from build123d import *

# Parameters (mm, degrees)
SKETCH_2_W                       = 1.5
SKETCH_2_H                       = 108.5
SM_BASE_FLANGE_1_DEPTH           = 385
SM_EDGE_FLANGE_2_STRIP_W         = 7.4732
SM_EDGE_FLANGE_2_STRIP_H         = 1.5
SM_EDGE_FLANGE_2_STRIP_CUT_DEPTH = 385
SM_EDGE_FLANGE_2_DEPTH           = 385
SKETCH_13_W                      = 19.831026495
SKETCH_13_H                      = 4.393295337
CUT_EXTRUDE_1_DEPTH              = 8
SM_EDGE_FLANGE_3_STRIP_W         = 7.4732
SM_EDGE_FLANGE_3_STRIP_H         = 1.5
SM_EDGE_FLANGE_3_STRIP_CUT_DEPTH = 385
SM_EDGE_FLANGE_3_DEPTH           = 385
SKETCH_18_W                      = 20.05650784
SKETCH_18_H                      = 5.183741357
CUT_EXTRUDE_2_DEPTH              = 8
SKETCH_19_W                      = 25.725423763
SKETCH_19_H                      = 11.342633063
CUT_EXTRUDE_3_DEPTH              = 140
SKETCH_20_W                      = 20.859346665
SKETCH_20_H                      = 6.188811882
CUT_EXTRUDE_4_DEPTH              = 15
SKETCH_21_W                      = 1.5
SKETCH_21_H                      = 153.4
EXTRUDE_1_DEPTH                  = 452.41
SKETCH_22_R                      = 2.75
CUT_EXTRUDE_5_DEPTH              = 20
SKETCH_23_R                      = 2.75
CUT_EXTRUDE_6_DEPTH              = 20
SKETCH_24_R                      = 2.75
CUT_EXTRUDE_7_DEPTH              = 20
SKETCH_28_W                      = 3.977690792
SKETCH_28_H                      = 20
CUT_EXTRUDE_8_DEPTH              = 10
SM_EDGE_FLANGE_5_STRIP_W         = 7.4732
SM_EDGE_FLANGE_5_STRIP_H         = 1.5
SM_EDGE_FLANGE_5_STRIP_CUT_DEPTH = 432.41
SM_EDGE_FLANGE_5_DEPTH           = 432.41
SKETCH_32_R                      = 2.75
CUT_EXTRUDE_9_DEPTH              = 10
CUT_EXTRUDE_START                = -2
CUT_EXTRUDE_10_DEPTH             = 2


# Read off the part's stored shape, not the designer's step: 切除-拉伸10
# Sheet-metal steps are written as plain solids
with BuildPart() as part:
    # Sketch 2 → 基体-法兰1 (new body)
    with BuildSketch(Plane.XY):
        with Locations((0.75, 54.25)):
            Rectangle(SKETCH_2_W, SKETCH_2_H)
    extrude(amount=SM_BASE_FLANGE_1_DEPTH)

    # 边线-法兰2 strip (across the edge) → 边线-法兰2 strip cut (cut)
    with BuildSketch(Plane(origin=(1.5, 0, 385), x_dir=(0, 1, 0), z_dir=(0, 0, -1))):
        with Locations((-1.5, -0.75)):
            Rectangle(SM_EDGE_FLANGE_2_STRIP_W, SM_EDGE_FLANGE_2_STRIP_H)
    extrude(amount=SM_EDGE_FLANGE_2_STRIP_CUT_DEPTH, mode=Mode.SUBTRACT)

    # 边线-法兰2 section (across the edge) → 边线-法兰2 (add)
    with BuildSketch(Plane(origin=(1.5, 0, 385), x_dir=(0, 1, 0), z_dir=(0, 0, -1))):
        with BuildLine():
            Line((0, 0.7366), (0, 13.5))
            Line((0, 13.5), (1.5, 13.5))
            Line((1.5, 13.5), (1.5, 0.7366))
            ThreePointArc((1.5, 0.7366), (1.715745145, 0.215745145), (2.2366, 0))
            Line((2.2366, 0), (2.2366, -1.5))
            ThreePointArc((2.2366, -1.5), (0.655084973, -0.844915027), (0, 0.7366))
        make_face()
    extrude(amount=SM_EDGE_FLANGE_2_DEPTH)

    # 草图13 → 切除-拉伸1 (cut)
    with BuildSketch(Plane(origin=(0, 0, 0), x_dir=(-1, 0, 0), z_dir=(0, 0, -1))):
        with Locations((-9.915513247, 0.039952332)):
            Rectangle(SKETCH_13_W, SKETCH_13_H)
    extrude(amount=-CUT_EXTRUDE_1_DEPTH, mode=Mode.SUBTRACT)

    # 边线-法兰3 strip (across the edge) → 边线-法兰3 strip cut (cut)
    with BuildSketch(Plane(origin=(1.5, 108.5, 0), x_dir=(0, -1, 0), z_dir=(0, 0, 1))):
        with Locations((-1.5, -0.75)):
            Rectangle(SM_EDGE_FLANGE_3_STRIP_W, SM_EDGE_FLANGE_3_STRIP_H)
    extrude(amount=SM_EDGE_FLANGE_3_STRIP_CUT_DEPTH, mode=Mode.SUBTRACT)

    # 边线-法兰3 section (across the edge) → 边线-法兰3 (add)
    with BuildSketch(Plane(origin=(1.5, 108.5, 0), x_dir=(0, -1, 0), z_dir=(0, 0, 1))):
        with BuildLine():
            Line((0, 0.7366), (0, 13.5))
            Line((0, 13.5), (1.5, 13.5))
            Line((1.5, 13.5), (1.5, 0.7366))
            ThreePointArc((1.5, 0.7366), (1.715745145, 0.215745145), (2.2366, 0))
            Line((2.2366, 0), (2.2366, -1.5))
            ThreePointArc((2.2366, -1.5), (0.655084973, -0.844915027), (0, 0.7366))
        make_face()
    extrude(amount=SM_EDGE_FLANGE_3_DEPTH)

    # 草图18 → 切除-拉伸2 (cut)
    with BuildSketch(Plane(origin=(0, 0, 0), x_dir=(-1, 0, 0), z_dir=(0, 0, -1))):
        with Locations((-10.02825392, 108.855270679)):
            Rectangle(SKETCH_18_W, SKETCH_18_H)
    extrude(amount=-CUT_EXTRUDE_2_DEPTH, mode=Mode.SUBTRACT)

    # 草图19 → 切除-拉伸3 (cut)
    with BuildSketch(Plane.XY.offset(385)):
        with Locations((12.862711882, 111.934716532)):
            Rectangle(SKETCH_19_W, SKETCH_19_H)
    extrude(amount=-CUT_EXTRUDE_3_DEPTH, mode=Mode.SUBTRACT)

    # 草图20 → 切除-拉伸4 (cut)
    with BuildSketch(Plane.XY.offset(245)):
        with Locations((10.429673333, 109.357805941)):
            Rectangle(SKETCH_20_W, SKETCH_20_H)
    extrude(amount=-CUT_EXTRUDE_4_DEPTH, mode=Mode.SUBTRACT)

    # 草图21 → 凸台-拉伸1 (add)
    with BuildSketch(Plane(origin=(0, 106.2634, 0), x_dir=(1, 0, 0), z_dir=(0, 1, 0))):
        with Locations((0.75, -308.3)):
            Rectangle(SKETCH_21_W, SKETCH_21_H)
    extrude(amount=EXTRUDE_1_DEPTH)

    # 草图22 → 切除-拉伸5 (cut)
    with BuildSketch(Plane.XZ.offset(-107)):
        with Locations((8.6183, 69)):
            Circle(SKETCH_22_R)
        with Locations((8.6183, 169)):
            Circle(SKETCH_22_R)
        with Locations((8.6183, 119)):
            Circle(SKETCH_22_R)
    extrude(amount=-CUT_EXTRUDE_5_DEPTH, mode=Mode.SUBTRACT)

    # 草图23 → 切除-拉伸6 (cut)
    with BuildSketch(Plane(origin=(0, 1.5, 0), x_dir=(1, 0, 0), z_dir=(0, 1, 0))):
        with Locations(Location((8.6183, -96.5, 0), (0, 0, 180))):
            Circle(SKETCH_23_R)
        with Locations(Location((8.6183, -196.5, 0), (0, 0, 180))):
            Circle(SKETCH_23_R)
        with Locations((8.6183, -296.5)):
            Circle(SKETCH_23_R)
    extrude(amount=-CUT_EXTRUDE_6_DEPTH, mode=Mode.SUBTRACT)

    # 草图24 → 切除-拉伸7 (cut)
    with BuildSketch(Plane(origin=(1.5, 0, 0), x_dir=(0, 0, -1), z_dir=(1, 0, 0))):
        with Locations((-377.815462169, 128.5882)):
            Circle(SKETCH_24_R)
        with Locations((-377.815462169, 278.5882)):
            Circle(SKETCH_24_R)
        with Locations((-377.815462169, 428.5882)):
            Circle(SKETCH_24_R)
    extrude(amount=-CUT_EXTRUDE_7_DEPTH, mode=Mode.SUBTRACT)

    # 草图28 → 切除-拉伸8 (cut)
    with BuildSketch(Plane(origin=(1.5, 0, 0), x_dir=(0, 0, -1), z_dir=(1, 0, 0))):
        with Locations((-233.588845396, 116.2634)):
            Rectangle(SKETCH_28_W, SKETCH_28_H)
    extrude(amount=-CUT_EXTRUDE_8_DEPTH, mode=Mode.SUBTRACT)

    # 边线-法兰5 strip (across the edge) → 边线-法兰5 strip cut (cut)
    with BuildSketch(Plane(origin=(1.5, 126.2634, 231.6), x_dir=(0, 0, 1), z_dir=(0, 1, 0))):
        with Locations((-1.5, -0.75)):
            Rectangle(SM_EDGE_FLANGE_5_STRIP_W, SM_EDGE_FLANGE_5_STRIP_H)
    extrude(amount=SM_EDGE_FLANGE_5_STRIP_CUT_DEPTH, mode=Mode.SUBTRACT)

    # 边线-法兰5 section (across the edge) → 边线-法兰5 (add)
    with BuildSketch(Plane(origin=(1.5, 126.2634, 231.6), x_dir=(0, 0, 1), z_dir=(0, 1, 0))):
        with BuildLine():
            Line((0, 0.7366), (0, 13.5))
            Line((0, 13.5), (1.5, 13.5))
            Line((1.5, 13.5), (1.5, 0.7366))
            ThreePointArc((1.5, 0.7366), (1.715745145, 0.215745145), (2.2366, 0))
            Line((2.2366, 0), (2.2366, -1.5))
            ThreePointArc((2.2366, -1.5), (0.655084973, -0.844915027), (0, 0.7366))
        make_face()
    extrude(amount=SM_EDGE_FLANGE_5_DEPTH)

    # 草图32 → 切除-拉伸9 (cut)
    with BuildSketch(Plane.XY.offset(233.1)):
        with Locations((8.6183, 462.4684)):
            Circle(SKETCH_32_R)
        with Locations((8.6183, 342.4684)):
            Circle(SKETCH_32_R)
        with Locations(Location((8.6183, 222.4684, 0), (0, 0, 180))):
            Circle(SKETCH_32_R)
    extrude(amount=-CUT_EXTRUDE_9_DEPTH, mode=Mode.SUBTRACT)

    # 切除-拉伸10 outline → 切除-拉伸10 (cut)
    with BuildSketch(Plane(origin=(0, 558.6734, 0), x_dir=(1, 0, 0), z_dir=(0, 1, 0)).offset(CUT_EXTRUDE_START)):
        with BuildLine():
            ThreePointArc((2.2366, -231.6), (0.655084973, -232.255084973), (0, -233.8366))
            Line((0, -233.8366), (1.5, -233.8366))
            ThreePointArc((1.5, -233.8366), (1.715745145, -233.315745145), (2.2366, -233.1))
            Line((2.2366, -233.1), (15, -233.1))
            Line((15, -233.1), (15, -231.6))
            Line((15, -231.6), (2.2366, -231.6))
        make_face()
    extrude(amount=CUT_EXTRUDE_10_DEPTH, mode=Mode.SUBTRACT)


solid = part.part
Geometry check sheet. Reference: the model listing, model coordinates, mm. A direction names the side the tool comes from. Round coordinates to 2 decimals unless told otherwise and drop trailing zeros. Order: outer loops, then holes, each group sorted by start corner. A loop starts at its lowest first (then second) coordinate and runs counter-clockwise, first axis right, second up. Notation, with made-up numbers: M 22,70.25 L 38,70.25 A15 ccw 38,74.25 Z; hole C -3.5,65 d5. An arc over 180 degrees is marked long. Write each question's results on one line, items separated by ' | '. Start each with the question number.
1. Material ranges on L1, parallel to Y at x = 12.75, z = 129; L2, parallel to X at y = 29, z = 44, recorded low to high. Write a range as from..to.
2. Cross-section at A-A on z = 80. Record the boundary of the cut face in (x, y), plus the area to 3 significant figures.
3. Set-up check for faces 4 (the face through (9, 338, 233.1)), 5 (the face through (1, 278, 385)), 6 (the face through (12, 107, 117)): record each of +Z, -Z, +X, -X, +Y, -Y from which the full face is reachable in a straight line by a thin tool's end or side.
4. Draft check along Y on faces 1 (the face through (9, 338, 231.6)), 2 (the face through (11, 108.5, 117)), 3 (the face through (1.5, 215, 281)). Enter one of: pulls with the +Y half, pulls with the -Y half, needs draft (parallel to the pull), parting line crosses it, or undercut.
5. Cross-section at C-C on x = 8.25. Give the number of separate pieces and of enclosed holes in the cut face, plus the area to 3 significant figures.
6. Go/stop test with flat-tipped pins: P1, Ø7, axis at x = 8.62, y = 222.47, coming from the +Z side; P2, Ø1, axis at x = 11.5, z = 52, coming from the +Y side; P3, Ø2.5, axis at x = 10, y = 1, coming from the -Z side. Record where each tip stops, or that it passes through.
7. Cross-section at B-B on y = 199. Record the boundary of the cut face in (x, z), plus the area to 3 significant figures.
Resolved:
1) L1: 0..1.5, 107..108.5 | L2: 0..1.5
2) outline: M 0,2.24 A2.24 ccw 2.24,0 L 15,0 L 15,1.5 L 2.24,1.5 A0.74 cw 1.5,2.24 L 1.5,106.26 A0.74 cw 2.24,107 L 15,107 L 15,108.5 L 2.24,108.5 A2.24 ccw 0,106.26 Z | area: 201 mm2
3) face 4: +Z, +X, +Y | face 5: +Z, +X, -X, +Y, -Y | face 6: +Z, -Z, +X
4) face 1: needs draft | face 2: pulls with the +Y half | face 3: undercut
5) separate pieces: 12 | enclosed holes: 0 | area: 1,470 mm2
6) P1: z = 233.1 | P2: y = 108.5 | P3: z = 8
7) outline: M 0,233.84 A2.24 ccw 2.24,231.6 L 15,231.6 L 15,233.1 L 2.24,233.1 A0.74 cw 1.5,233.84 L 1.5,385 L 0,385 Z | area: 249 mm2
